Work out the finished part from the listing and answer in its coordinate system (mm). Give positions to 0.01 mm unless a question says otherwise; leave off trailing zeros. Loops run counter-clockwise (first coordinate to the right, second up) from the corner with the lowest first, then second, coordinate; pieces in that order, holes last. Notation, with made-up numbers: (80, -27) -> (92, -27) arc R32 ccw to (92, 3) -> close; hole circle Ø8 at (-15.75, -23.5). An arc over 180 degrees is marked (long way). Answer as CSV lines item,"result". Start each with the question number.
1. Find section A-A, the plane x = 58. Give the vertices of the cut face in (y, z).
2. Find section C-C, the plane x = -4.5. Give the vertices of the cut face in (y, z), and give its area (3 significant figures).
3. Flat-ended cylindrical pins translate along their axes: pin 1 Ø2.5 at (x, y) = (217, 461.5) entering from +Z; pin 2 Ø2.5 at (y, z) = (461.5, 51) entering from -X; pin 3 Ø2.5 at (x, y) = (-166.5, 462) entering from +Z. Find the tip coordinate at first contact, or state that the pin passes through.
4. Find section B-B, the plane y = 463. Count the separate pieces of the cut face and the enclosed holes in it, and give its area (3 significant figures).
5. Find the intervals of material crossed by line 1 along X through (y, z) = (463.25, -10); line 2 along X through (y, z) = (463.5, 31); line 3 along Z through (x, y) = (-140, 462.95), in increasing order.
from build123d import *

# Parameters (mm, degrees)
STOCK_FRAME_START              = 460
STOCK_FRAME_MASTER_1_OUTLINE_R = 2
STOCK_FRAME_MASTER_1_DEPTH     = 5
SKETCH4_R                      = 2
CUT_EXTRUDE3_DEPTH             = 262.655447486
SKETCH1_R                      = 2.5
CUT_EXTRUDE1_DEPTH             = 313.332847009
SKETCH2_W                      = 5
SKETCH2_H                      = 2
CUT_EXTRUDE2_DEPTH             = 313.332847009


# Read off the part's stored shape, not the designer's step: Stock-Frame master-1
with BuildPart() as part:
    # Stock-Frame master-1 outline → Stock-Frame master-1 (new body)
    with BuildSketch(Plane(origin=(0, 0, 0), x_dir=(1, 0, 0), z_dir=(0, 1, 0)).offset(STOCK_FRAME_START)):
        with BuildLine():
            Line((220, 51.342522712), (220, 57.685045424))
            ThreePointArc((220, 57.685045424), (217.722431864, 66.185045424), (211.5, 72.407477288))
            Line((211.5, 72.407477288), (138.354945114, 114.637794416))
            Line((138.354945114, 114.637794416), (135.854945114, 110.307667397))
            Line((135.854945114, 110.307667397), (114.20431002, 122.807667397))
            Line((114.20431002, 122.807667397), (116.70431002, 127.137794416))
            Line((116.70431002, 127.137794416), (95.053674925, 139.637794416))
            Line((95.053674925, 139.637794416), (92.553674925, 135.307667397))
            Line((92.553674925, 135.307667397), (81.728357378, 141.557667397))
            Line((81.728357378, 141.557667397), (0, 0))
            Line((0, 0), (220, 0))
            Line((220, 0), (220, 6.342522712))
            Line((220, 6.342522712), (215, 6.342522712))
            Line((215, 6.342522712), (215, 21.342522712))
            Line((215, 21.342522712), (220, 21.342522712))
            Line((220, 21.342522712), (220, 36.342522712))
            Line((220, 36.342522712), (215, 36.342522712))
            Line((215, 36.342522712), (215, 51.342522712))
            Line((215, 51.342522712), (220, 51.342522712))
        make_face()
        with Locations((188.660254038, 62.5)):
            Circle(STOCK_FRAME_MASTER_1_OUTLINE_R, mode=Mode.SUBTRACT)
        with Locations((171.339745962, 72.5)):
            Circle(STOCK_FRAME_MASTER_1_OUTLINE_R, mode=Mode.SUBTRACT)
    extrude(amount=STOCK_FRAME_MASTER_1_DEPTH)

    # Sketch4 → Cut-Extrude3 (cut, through all)
    with BuildSketch(Plane(origin=(0, 465, 0), x_dir=(1, 0, 0), z_dir=(0, 1, 0))):
        with Locations(Location((200, 31, 0), (0, 0, 270))):
            Circle(SKETCH4_R)
    extrude(amount=-CUT_EXTRUDE3_DEPTH, mode=Mode.SUBTRACT)

    # Mirror1: part across plane


with BuildPart() as part_1:
    add(part.part)
    add(part.part.mirror(Plane(origin=(0, 465, 0), x_dir=(1, 0, 0), z_dir=(0, 0, -1))))


with BuildPart() as body_2:
    # Mirror2: mirrored copy
    add(part_1.part.mirror(Plane(origin=(81.728357378, 465, -141.557667397), x_dir=(-0.49999999999999395, 0, 0.866025403784442), z_dir=(0.8660254037844421, 0, 0.49999999999999395))))


with BuildPart() as body_3:
    # Mirror3: mirrored copy
    add(part_1.part.mirror(Plane(origin=(81.728357378, 465, 141.557667397), x_dir=(0.49999999999999395, 0, 0.866025403784442), z_dir=(0.8660254037844421, 0, -0.49999999999999395))))

    # Combine1: union body 2, part
    add(body_2.part)
    add(part_1.part)

    # Sketch1 → Cut-Extrude1 (cut, through all)
    with BuildSketch(Plane(origin=(0, 465, 0), x_dir=(1, 0, 0), z_dir=(0, 1, 0))):
        with Locations(Location((25, 10, 0), (0, 0, 270))):
            Circle(SKETCH1_R)
        with Locations(Location((25, -10, 0), (0, 0, 270))):
            Circle(SKETCH1_R)
    extrude(amount=-CUT_EXTRUDE1_DEPTH, mode=Mode.SUBTRACT)

    # Sketch2 → Cut-Extrude2 (cut, through all)
    with BuildSketch(Plane(origin=(0, 465, 0), x_dir=(1, 0, 0), z_dir=(0, 1, 0))):
        with Locations((42.5, 6)):
            Rectangle(SKETCH2_W, SKETCH2_H)
        with Locations((42.5, -6)):
            Rectangle(SKETCH2_W, SKETCH2_H)
        with Locations((162.5, 6)):
            Rectangle(SKETCH2_W, SKETCH2_H)
        with Locations((162.5, -6)):
            Rectangle(SKETCH2_W, SKETCH2_H)
    extrude(amount=-CUT_EXTRUDE2_DEPTH, mode=Mode.SUBTRACT)


solid = body_3.part
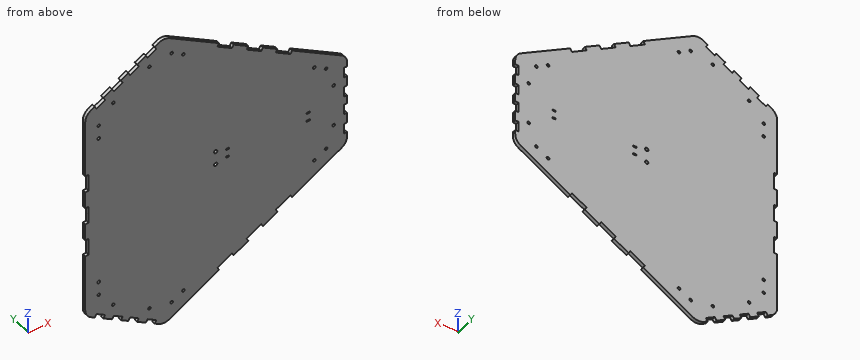
Resolved:
1,outline,"(460, -161.03) -> (465, -161.03) -> (465, 161.03) -> (460, 161.03) -> close"
2,outline,"(460, -197.12) -> (465, -197.12) -> (465, 197.12) -> (460, 197.12) -> close"
2,area,"1,970 mm^2"
3,pin 1,"stops at z = 68.93"
3,pin 2,"stops at x = -163.46"
3,pin 3,"stops at z = 156.9"
4,separate pieces,"1"
4,enclosed holes,"24"
4,area,"121,000 mm^2"
5,line 1,"x = -163.46 to 22.5, 27.5 to 215"
5,line 2,"x = -168.46 to 198, 202 to 220"
5,line 3,"z = -173.21 to -169.8, -167.43 to 167.43, 169.8 to 173.21"
